Geometry check sheet. Reference: the model listing, model coordinates, mm. Face numbers are marked on the shaded views. A direction names the side the tool comes from. Give positions to 0.01 mm unless a question says otherwise; leave off trailing zeros. Loops run counter-clockwise (first coordinate to the right, second up) from the corner with the lowest first, then second, coordinate; pieces in that order, holes last. Notation, with made-up numbers: (-0.75, 71.25) -> (49.25, 71.25) arc R8 cw to (49.25, 79.25) -> close; hole circle Ø9 at (7, 66.5). An arc over 180 degrees is marked (long way). Write each question's results on one line, items separated by ' | '. Start each with the question number.
1) Depth check by flat-ended pin: pin 1 (6.5 mm diameter, centred on y = -7.5, z = 0, fed in from +X); pin 2 (6 mm diameter, centred on x = 4, z = 4.5, fed in from -Y); pin 3 (8 mm diameter, centred on x = -3.5, y = -7, fed in from +Z); pin 4 (3 mm diameter, centred on x = 4.5, z = -4, fed in from -Y). Enter the tip coordinate at first touch or a pass-through.
2) Set-up check for the marked faces 1, 2 and 3: record each of +Z, -Z, +X, -X, +Y, -Y from which the full face is reachable in a straight line by a thin tool's end or side.
3) Scan lines: line 1 (Y direction, x = 0.5, z = -4); line 2 (Y direction, x = 0.75, z = 1); line 3 (X direction, y = -8.5, z = -4). Record each from-to range of solid material in increasing order. Write a range as from..to.
4) Draft check along Y on the marked faces 4, 5 and 6. Enter one of: pulls with the +Y half, pulls with the -Y half, needs draft (parallel to the pull), parting line crosses it, or undercut.
5) Sectioned sample at D-D on y = -13.5. Record the cut outline in (x, z).
6) Sectioned sample at A-A on x = -1.5. Count the separate pieces of the cut face and the enclosed holes in it, then the cut area to 3 significant figures.
Solid Edge part; units mm, degrees
sketch "Sketch1" plane through (0, 0, 0) normal (0, -1, 0) x (1, 0, 0)
  line L0 (-7.5, -7.5) -> (7.5, -7.5)
  line L1 (7.5, -7.5) -> (7.5, 7.5)
  line L2 (7.5, 7.5) -> (-7.5, 7.5)
  line L3 (-7.5, 7.5) -> (-7.5, -7.5)
  dimension "D1" = 7.5
  dimension "D2" = 7.5
extrude "Protrusion1" add sketch "Sketch1" along normal blind 40
sketch "Sketch2" plane through (7.5, -20, 0) normal (1, 0, 0) x (0, 1, 0)
  line L0 (-20, 7.5) -> (-3, 7.5)
  line L1 (-3, 7.5) -> (-3, 0)
  line L2 (-3, 0) -> (-20, 0)
  line L3 (-20, 0) -> (-20, 7.5)
  dimension "D1" = 20
extrude "Cutout1" cut sketch "Sketch2" against normal through all
sketch "Sketch3" plane through (0, -11.5, 7.5) normal (0, 0, 1) x (1, 0, 0)
  line L0 (7.5, 11.5) -> (0, 11.5)
  line L1 (0, 11.5) -> (0, -6)
  line L2 (0, -6) -> (7.5, -6)
  line L3 (7.5, -6) -> (7.5, 11.5)
  dimension "D1" = 7.5
extrude "Cutout2" cut sketch "Sketch3" against normal through all
fillet "Verrundung_1" radius 7.5 4 edges at (7.5, -40, -3.75) (-7.5, -40, -3.75) (-3.75, 0, 7.5) (-3.75, 0, -7.5)
sketch "Sketch4" plane through (0, -8.75, 0) normal (1, 0, 0) x (0, 0, -1)
  circle A0 centre (0, 1.25) radius 2.05
extrude "Cutout3" cut sketch "Sketch4" against normal through all
sketch "Sketch5" plane through (0, -31.5, 0) normal (0, 0, 1) x (1, 0, 0)
  circle A0 centre (0, -1) radius 2.05
extrude "Cutout4" cut sketch "Sketch5" against normal through all
chamfer "Fase_1" distance 1 angle 45 4 edges at (0, -7.5, 2.05) (-2.05, -32.5, 0) (-2.05, -32.5, -7.5) (-7.5, -7.5, 2.05)
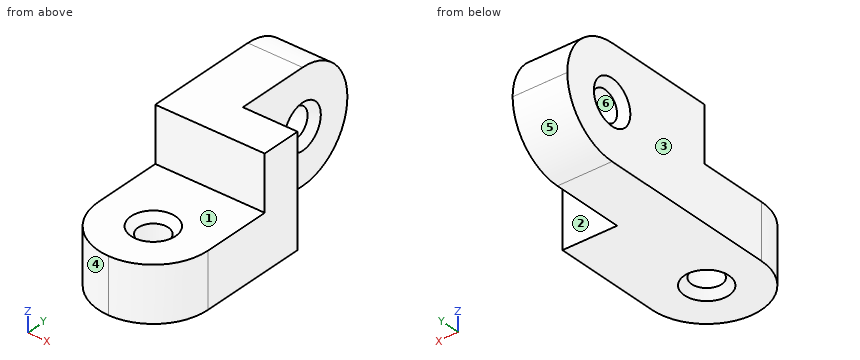
Result:
1) pin 1: x = 0 | pin 2: y = -23 | pin 3: z = 7.5 | pin 4: y = -39.37
2) face 1: +Z, +X, -X, -Y | face 2: +Z, -Z, +X, +Y | face 3: +Z, -Z, -X, +Y, -Y
3) line 1: -39.98..-34.49, -30.51..-17.5 | line 2: -23..-17.5 | line 3: -7.5..0
4) face 4: pulls with the -Y half | face 5: pulls with the +Y half | face 6: undercut
5) outline: (-7.5, -7.5) -> (0, -7.5) -> (0, 7.5) -> (-7.5, 7.5) -> close
6) separate pieces: 2 | enclosed holes: 1 | area: 410 mm^2
